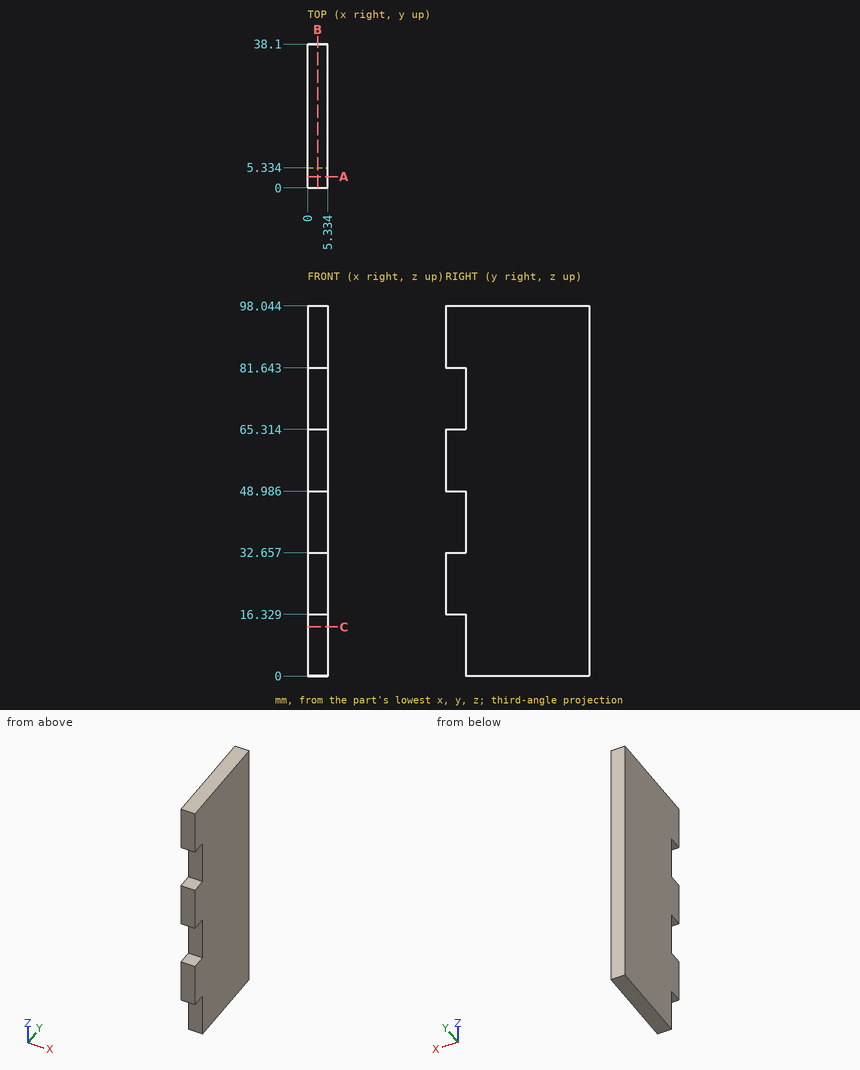
Geometry check sheet. Reference: drawing and pictorial views, mm from the part's lowest x, y, z. Coordinates: 2 decimals unless noted, no trailing zeros. Write each loop counter-clockwise with the first axis right and the second up, starting at its lowest first coordinate (ties: lowest second). Pieces come first, ordered by that corner, then holes.
Item 1: Scan lines: probe 1 along Z at (x, y) = (2.95, 2.5) (1 decimal); probe 2 along Y at (x, z) = (1.5, 41.5). Record each from-to range of solid material in increasing order.
Numbers:
probe 1: z = 16.3 to 32.7, 49 to 65.3, 81.6 to 98
probe 2: y = 5.33 to 38.1
Item 2: Cross-section at C-C on z = 13. Record the boundary of the cut face in (x, y), then the cut area to 3 significant figures.
Numbers:
outline: (0, 5.33) - (5.33, 5.33) - (5.33, 38.1) - (0, 38.1) - close
area: 175 mm2
Item 3: Cross-section at A-A on y = 3. Record the boundary of the cut face in (x, z) (1 decimal).
Numbers:
outline: (0, 16.3) - (5.3, 16.3) - (5.3, 32.7) - (0, 32.7) - close; (0, 49) - (5.3, 49) - (5.3, 65.3) - (0, 65.3) - close; (0, 81.6) - (5.3, 81.6) - (5.3, 98) - (0, 98) - close
Item 4: Depth check by flat-ended pin: pin 1 Ø2.5 at (x, z) = (2.5, 39.5) entering from -Y; pin 2 Ø1.6 at (x, y) = (3, 2.5) entering from -Z. Enter the tip coordinate at first touch or a pass-through.
Numbers:
pin 1: stops at y = 5.33
pin 2: stops at z = 16.33
Item 5: Cross-section at B-B on x = 2.7. Record the boundary of the cut face in (y, z) (1 decimal), then the cut area to 3 significant figures.
Numbers:
outline: (0, 16.3) - (5.3, 16.3) - (5.3, 0) - (38.1, 0) - (38.1, 98) - (0, 98) - (0, 81.6) - (5.3, 81.6) - (5.3, 65.3) - (0, 65.3) - (0, 49) - (5.3, 49) - (5.3, 32.7) - (0, 32.7) - close
area: 3,470 mm2
